Could you check a few things on this model? Use its own coordinates, in mm. A direction names the side the tool comes from. Give positions to 0.01 mm unless a question says otherwise; leave off trailing zeros. Order: outer loops, then holes, each group sorted by start corner. A loop starts at its lowest first (then second) coordinate and runs counter-clockwise, first axis right, second up.
from build123d import *

# Parameters (mm, degrees)
SKETCH1_W                 = 70
SKETCH1_H                 = 15
BOSS_EXTRUDE1_DEPTH       = 5
SKETCH3_W                 = 5
SKETCH3_H                 = 15
BOSS_EXTRUDE2_DEPTH       = 45
F_6_0MM_DOWEL_HOLE1_D     = 6
F_6_0MM_DOWEL_SLOT1_DEPTH = 5
BOSS_EXTRUDE3_DEPTH       = 50.83
F_6_0MM_DOWEL_SLOT2_DEPTH = 5
F_6_0MM_DOWEL_HOLE2_D     = 6
F_6_0MM_DOWEL_HOLE2_DEPTH = 7.999
F_6_0MM_DOWEL_HOLE2_TIP   = 1.802581857
BOSS_EXTRUDE4_DEPTH       = 5
BOSS_EXTRUDE5_DEPTH       = 5
SKETCH19_W                = 5
SKETCH19_H                = 75.83
BOSS_EXTRUDE6_DEPTH       = 11.3
SKETCH20_W                = 75.83
SKETCH20_H                = 5
BOSS_EXTRUDE7_DEPTH       = 35
F_6_0MM_START             = -11.3
F_6_0MM_DOWEL_SLOT3_DEPTH = 5


# Read off the part's stored shape, not the designer's step: Ø6.0mm Dowel Slot1, Ø6.0mm Dowel Slot2, Ø6.0mm Dowel Slot3
with BuildPart() as part:
    # Sketch1 → Boss-Extrude1 (new body)
    with BuildSketch(Plane(origin=(0, 0, 0), x_dir=(1, 0, 0), z_dir=(0, 1, 0))):
        with Locations((4.827783478, -3.453636176)):
            Rectangle(SKETCH1_W, SKETCH1_H)
    extrude(amount=BOSS_EXTRUDE1_DEPTH)

    # Sketch3 → Boss-Extrude2 (add)
    with BuildSketch(Plane(origin=(0, 5, 0), x_dir=(1, 0, 0), z_dir=(0, 1, 0))):
        with Locations((-27.672216522, -3.453636176)):
            Rectangle(SKETCH3_W, SKETCH3_H)
    extrude(amount=BOSS_EXTRUDE2_DEPTH)

    # Ø6.0mm Dowel Hole1 (through all)
    with Locations(Plane.ZY.offset(30.172216522)):
        with Locations((3.453636176, 15), (3.453636176, 40)):
            Hole(F_6_0MM_DOWEL_HOLE1_D / 2)

    # Ø6.0mm Dowel Slot1 outline → Ø6.0mm Dowel Slot1 (cut)
    with BuildSketch(Plane(origin=(0, 0, 0), x_dir=(1, 0, 0), z_dir=(0, 1, 0))):
        with BuildLine():
            Line((19.509331286, -6.453444287), (29.209331286, -6.453444287))
            ThreePointArc((29.209331286, -6.453444287), (32.209331286, -3.453444287), (29.209331286, -0.453444287))
            Line((29.209331286, -0.453444287), (19.509331286, -0.453444287))
            ThreePointArc((19.509331286, -0.453444287), (16.509331286, -3.453444287), (19.509331286, -6.453444287))
        make_face()
        with BuildLine():
            Line((-12.530668714, -6.453557031), (-2.830668714, -6.453557031))
            ThreePointArc((-2.830668714, -6.453557031), (0.169331286, -3.453557031), (-2.830668714, -0.453557031))
            Line((-2.830668714, -0.453557031), (-12.530668714, -0.453557031))
            ThreePointArc((-12.530668714, -0.453557031), (-15.530668714, -3.453557031), (-12.530668714, -6.453557031))
        make_face()
    extrude(amount=F_6_0MM_DOWEL_SLOT1_DEPTH, mode=Mode.SUBTRACT)

    # Sketch10 → Boss-Extrude3 (add)
    with BuildSketch(Plane(origin=(0, 0, -4.046363824), x_dir=(-1, 0, 0), z_dir=(0, 0, -1))):
        Polygon((-39.827783478, 5), (-39.827783478, 0), (30.172216522, 0), (30.172216522, 50), (25.172216522, 50), (25.172216522, 5), align=None)
    extrude(amount=BOSS_EXTRUDE3_DEPTH)

    # Ø6.0mm Dowel Slot2 outline → Ø6.0mm Dowel Slot2 (cut)
    with BuildSketch(Plane(origin=(0, 0, 0), x_dir=(1, 0, 0), z_dir=(0, 1, 0))):
        with BuildLine():
            Line((19.509331286, 44.376555713), (29.209331286, 44.376555713))
            ThreePointArc((29.209331286, 44.376555713), (32.209331286, 47.376555713), (29.209331286, 50.376555713))
            Line((29.209331286, 50.376555713), (19.509331286, 50.376555713))
            ThreePointArc((19.509331286, 50.376555713), (16.509331286, 47.376555713), (19.509331286, 44.376555713))
        make_face()
        with BuildLine():
            Line((-12.530668714, 44.376442969), (-2.830668714, 44.376442969))
            ThreePointArc((-2.830668714, 44.376442969), (0.169331286, 47.376442969), (-2.830668714, 50.376442969))
            Line((-2.830668714, 50.376442969), (-12.530668714, 50.376442969))
            ThreePointArc((-12.530668714, 50.376442969), (-15.530668714, 47.376442969), (-12.530668714, 44.376442969))
        make_face()
    extrude(amount=F_6_0MM_DOWEL_SLOT2_DEPTH, mode=Mode.SUBTRACT)

    # Ø6.0mm Dowel Hole2
    with Locations(Plane(origin=(-25.172216522, 0, 0), x_dir=(0, 0, -1), z_dir=(1, 0, 0))):
        with Locations((47.376442969, 40), (47.376442969, 15)):
            Hole(F_6_0MM_DOWEL_HOLE2_D / 2, depth=F_6_0MM_DOWEL_HOLE2_DEPTH)
            with Locations((0, 0, -(F_6_0MM_DOWEL_HOLE2_DEPTH + F_6_0MM_DOWEL_HOLE2_TIP / 2))):  # 118° drill point
                Cone(0, F_6_0MM_DOWEL_HOLE2_D / 2, F_6_0MM_DOWEL_HOLE2_TIP, mode=Mode.SUBTRACT)

    # Sketch17 → Boss-Extrude4 (add)
    with BuildSketch(Plane.XY.offset(10.953636176)):
        Polygon((-25.172216522, 50), (7.327783478, 5), (39.827783478, 5), (39.827783478, 0), (7.327783478, 0), (-30.172216522, 0), (-30.172216522, 50), align=None)
    extrude(amount=BOSS_EXTRUDE4_DEPTH)

    # Sketch18 → Boss-Extrude5 (add)
    with BuildSketch(Plane(origin=(0, 0, -54.876363824), x_dir=(-1, 0, 0), z_dir=(0, 0, -1))):
        Polygon((25.172216522, 50), (-7.327783478, 5), (-39.827783478, 5), (-39.827783478, 0), (30.172216522, 0), (30.172216522, 50), align=None)
    extrude(amount=BOSS_EXTRUDE5_DEPTH)

    # Sketch19 → Boss-Extrude6 (add)
    with BuildSketch(Plane.XZ):
        with Locations((-27.672216522, -21.961363824)):
            Rectangle(SKETCH19_W, SKETCH19_H)
    extrude(amount=BOSS_EXTRUDE6_DEPTH)

    # Sketch20 → Boss-Extrude7 (add)
    with BuildSketch(Plane(origin=(-25.172216522, 0, 0), x_dir=(0, 0, -1), z_dir=(1, 0, 0))):
        with Locations((21.961363824, -8.8)):
            Rectangle(SKETCH20_W, SKETCH20_H)
    extrude(amount=BOSS_EXTRUDE7_DEPTH)

    # Ø6.0mm Dowel Slot3 outline → Ø6.0mm Dowel Slot3 (cut)
    with BuildSketch(Plane(origin=(0, 0, 0), x_dir=(1, 0, 0), z_dir=(0, 1, 0)).offset(F_6_0MM_START)):
        with BuildLine():
            Line((-12.530668714, -6.453557031), (-2.830668714, -6.453557031))
            ThreePointArc((-2.830668714, -6.453557031), (0.169331286, -3.453557031), (-2.830668714, -0.453557031))
            Line((-2.830668714, -0.453557031), (-12.530668714, -0.453557031))
            ThreePointArc((-12.530668714, -0.453557031), (-15.530668714, -3.453557031), (-12.530668714, -6.453557031))
        make_face()
        with BuildLine():
            Line((-12.530668714, 44.376442969), (-2.830668714, 44.376442969))
            ThreePointArc((-2.830668714, 44.376442969), (0.169331286, 47.376442969), (-2.830668714, 50.376442969))
            Line((-2.830668714, 50.376442969), (-12.530668714, 50.376442969))
            ThreePointArc((-12.530668714, 50.376442969), (-15.530668714, 47.376442969), (-12.530668714, 44.376442969))
        make_face()
    extrude(amount=F_6_0MM_DOWEL_SLOT3_DEPTH, mode=Mode.SUBTRACT)


solid = part.part
Item 1: Imagine slicing it at B-B on y = 40. List the corners of the cut face in (x, z) for me, then the cut area to 3 significant figures.
Findings:
outline: (-30.17, -59.88) - (-17.95, -59.88) - (-17.95, -54.88) - (-25.17, -54.88) - (-25.17, -50.38) - (-30.17, -50.38) - close; (-30.17, -44.38) - (-25.17, -44.38) - (-25.17, 0.45) - (-30.17, 0.45) - close; (-30.17, 6.45) - (-25.17, 6.45) - (-25.17, 10.95) - (-17.95, 10.95) - (-17.95, 15.95) - (-30.17, 15.95) - close
area: 391 mm2
Item 2: Imagine slicing it at C-C on x = -11.5. List the corners of the cut face in (y, z) for me, then the cut area to 3 significant figures.
Findings:
outline: (-11.3, -59.88) - (-6.3, -59.88) - (-6.3, -50.38) - (-11.3, -50.38) - close; (-11.3, -44.38) - (-6.3, -44.38) - (-6.3, 0.45) - (-11.3, 0.45) - close; (-11.3, 6.45) - (-6.3, 6.45) - (-6.3, 15.95) - (-11.3, 15.95) - close; (0, -59.88) - (31.07, -59.88) - (31.07, -54.88) - (5, -54.88) - (5, -50.38) - (0, -50.38) - close; (0, -44.38) - (5, -44.38) - (5, 0.45) - (0, 0.45) - close; (0, 6.45) - (5, 6.45) - (5, 10.95) - (31.07, 10.95) - (31.07, 15.95) - (0, 15.95) - close
area: 899 mm2
Item 3: We'd pull the mould along Z, two halves only. Please class faces 1 (the cylindrical face through (32.21, 2.46, -47.31)), 2 (the flat face through (-11, 12, 15.954)), 3 (the flat face through (9.828, -9, -21)): +Z half, -Z half, draft (parallel to the pull), parting line (faces both ways), or undercut.
Findings:
face 1: undercut
face 2: +Z half
face 3: draft
Item 4: Imagine slicing it at A-A on x = 24.5. List the corners of the cut face in (y, z) for me, then the cut area to 3 significant figures.
Findings:
outline: (0, -59.88) - (5, -59.88) - (5, -50.38) - (0, -50.38) - close; (0, -44.38) - (5, -44.38) - (5, 0.45) - (0, 0.45) - close; (0, 6.45) - (5, 6.45) - (5, 15.95) - (0, 15.95) - close
area: 319 mm2
Item 5: Imagine slicing it at D-D on z = 3.5. Give the number of separate pieces and of enclosed holes in the cut face, then the cut area to 3 significant figures.
Findings:
separate pieces: 6
enclosed holes: 0
area: 511 mm2
Item 6: Please list where these lines run through material, in increasing order: line 1 along Z through (x, y) = (-19.5, 16.5); line 2 along Y through (x, z) = (-23.5, -29.5); line 3 along Z through (x, y) = (-27, 41.5).
Findings:
line 1: z = -59.88 to -54.88, 10.95 to 15.95
line 2: y = -11.3 to -6.3, 0 to 5
line 3: z = -59.88 to -49.97, -44.78 to 0.86, 6.05 to 15.95
Item 7: For pin 1 (7 mm diameter, centred on y = 15, z = 3.45, fed in from +X); pin 2 (10 mm diameter, centred on x = 11, z = -31.5, fed in from +Y); pin 3 (12 mm diameter, centred on x = -10, y = -2, fed in from +Z); pin 4 (10 mm diameter, centred on x = 15.5, z = -25.5, fed in from -Y), each with a flat end and sliding along its axis, tell me the tip position at first contact or that it passes through.
Findings:
pin 1: stops at x = -25.17
pin 2: stops at y = 5
pin 3: stops at z = 15.95
pin 4: stops at y = 0
Item 8: For faces 4 (the flat face through (-8, -9, -44.376)), 5 (the cylindrical face through (-27.64, 12.07, 4.1)), 6 (the flat face through (-25.172, 28, -22)), which set-ups out of +Z, -Z, +X, -X, +Y, -Y let a thin tool reach every point of the face, with its end or its side?
Findings:
face 4: +Y, -Y
face 5: +X, -X
face 6: +X, +Y
